Check sheet for the modelled part. Datum: model origin and axes. Units: mm. Face numbers are marked on the shaded views. A direction names the side the tool comes from. Give positions to 0.01 mm unless a question says otherwise; leave off trailing zeros. Order: outer loops, then holes, each group sorted by start corner. A loop starts at its lowest first (then second) coordinate and runs counter-clockwise, first axis right, second up. Notation, with made-up numbers: M -30.75,27 L -10.75,27 A21 cw -10.75,51 Z; hole C -17.5,-29.75 d2. An arc over 180 degrees is marked long. One line per question, with ' | ' between items. Start each with the question number.
```python
from build123d import *

# Parameters (mm, degrees)
BOSS_EXTRUDE1_DEPTH   = 19.812
SKETCH2_R             = 7.62
BOSS_EXTRUDE2_DEPTH   = 14.986
BOSS_EXTRUDE3_DEPTH   = 19.812
CHAMFER1_SIZE2        = 1.397459912
CHAMFER1_SIZE         = 1.361150227
CHAMFER1_EDGE_2_SIZE2 = 1.397459912
CHAMFER1_EDGE_2_SIZE  = 1.361150227


with BuildPart() as part:
    # Sketch1 → Boss-Extrude1 (new body)
    with BuildSketch(Plane(origin=(0, 0, 0), x_dir=(0, -1, 0), z_dir=(-1, 0, 0))):
        Polygon((-9.525, 5.499261314), (-9.525, -5.499261314), (0, -10.998522628), (9.525, -5.499261314), (9.525, 5.499261314), (0, 10.998522628), align=None)
    extrude(amount=-BOSS_EXTRUDE1_DEPTH)

    # Sketch2 → Boss-Extrude2 (add)
    with BuildSketch(Plane(origin=(19.812, 0, 0), x_dir=(0, 0, -1), z_dir=(1, 0, 0))):
        Circle(SKETCH2_R)
    extrude(amount=BOSS_EXTRUDE2_DEPTH)

    # Sketch3 → Boss-Extrude3 (add)
    with BuildSketch(Plane(origin=(34.798, 0, 0), x_dir=(0, -1, 0), z_dir=(-1, 0, 0))):
        Polygon((9.525, -5.499261314), (9.525, 5.499261314), (0, 10.998522628), (-9.525, 5.499261314), (-9.525, -5.499261314), (0, -10.998522628), align=None)
    extrude(amount=-BOSS_EXTRUDE3_DEPTH)

    # Sketch4 → Hole1 (revolve, cut)
    with BuildSketch(Plane(origin=(54.61, 0, 0), x_dir=(0, 0, -1), z_dir=(0, 1, 0))):
        Polygon((0, 0), (0, 9.906), (5.49664229, 9.906), (5.750849773, 0), align=None)
    revolve(axis=Axis((-55.39, 0, 0), (1, 0, 0)), mode=Mode.SUBTRACT)

    # Sketch6 → Hole2 (revolve, cut)
    with BuildSketch(Plane.ZX):
        Polygon((0, 0), (0, 9.906), (5.49664229, 9.906), (5.750849773, 0), align=None)
    revolve(axis=Axis((110, 0, 0), (-1, 0, 0)), mode=Mode.SUBTRACT)

    # Chamfer1
    chamfer1_edges = [part.edges().sort_by_distance(p)[0] for p in [
        (54.61, 0, 5.750849773),
    ]]
    chamfer(chamfer1_edges, length=CHAMFER1_SIZE, length2=CHAMFER1_SIZE2)

    # Chamfer1 edge 2
    chamfer1_edge_2_edges = [part.edges().sort_by_distance(p)[0] for p in [
        (0, 0, -5.750849773),
    ]]
    chamfer(chamfer1_edge_2_edges, length=CHAMFER1_EDGE_2_SIZE, length2=CHAMFER1_EDGE_2_SIZE2)


solid = part.part
```
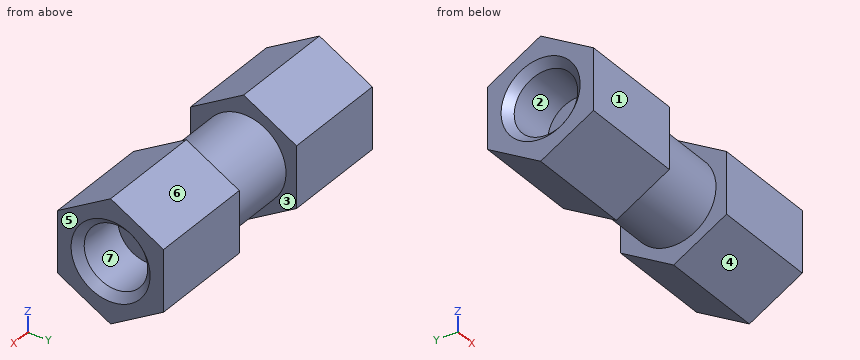
Item 1: Set-up check for the marked faces 1, 2 and 3: record each of +Z, -Z, +X, -X, +Y, -Y from which the full face is reachable in a straight line by a thin tool's end or side.
Item 2: Draft check along Z on the marked faces 4, 5, 6 and 7. Enter one of: released by +Z, released by -Z, zero draft, split by the parting line, or undercut.
Item 3: Go/stop test with flat-tipped pins: P1, Ø9, axis at y = -1.5, z = 1, coming from the -X side; P2, Ø3.5, axis at y = -0.5, z = 2, coming from the +X side; P3, Ø1.5, axis at x = 23.5, y = -3, coming from the -Z side. Record where each tip stops, or that it passes through.
Item 4: Section check D-D, the plane z = 8.5. Record the cut outline in (x, y).
Item 5: Section check A-A, the plane z = 0. Record the cut outline in (x, y) (3 decimals), then the cut area to 3 significant figures.
Item 6: Scan lines: probe 1 along X at (y, z) = (1.5, 10); probe 2 along Y at (x, z) = (47, -0.75) (3 decimals); probe 3 along Z at (x, y) = (51, 1). Record each from-to range of solid material in increasing order. Write a range as [from, to].
Item 7: Section check B-B, the plane y = 8.25. Record the cut outline in (x, z), then the cut area to 3 significant figures.
Item 8: Section check C-C, the plane x = 17. Record the cut outline in (y, z) (3 decimals).
Reported:
1) face 1: +Z, -Z, +X, -X, -Y | face 2: -X | face 3: none
2) face 4: released by -Z | face 5: zero draft | face 6: released by +Z | face 7: undercut
3) P1: stops at x = 0.81 | P2: stops at x = 44.7 | P3: stops at z = -7.28
4) outline: M 0,-4.33 L 19.81,-4.33 L 19.81,4.33 L 0,4.33 Z; M 34.8,-4.33 L 54.61,-4.33 L 54.61,4.33 L 34.8,4.33 Z
5) outline: M 0,-9.525 L 19.812,-9.525 L 19.812,-7.62 L 34.798,-7.62 L 34.798,-9.525 L 54.61,-9.525 L 54.61,-7.112 L 53.213,-5.715 L 44.704,-5.497 L 44.704,5.497 L 53.213,5.715 L 54.61,7.112 L 54.61,9.525 L 34.798,9.525 L 34.798,7.62 L 19.812,7.62 L 19.812,9.525 L 0,9.525 L 0,7.112 L 1.397,5.715 L 9.906,5.497 L 9.906,-5.497 L 1.397,-5.715 L 0,-7.112 Z | area: 757 mm^2
6) probe 1: x = [0, 19.81], [34.8, 54.61] | probe 2: y = [-9.525, -5.505], [5.505, 9.525] | probe 3: z = [-10.42, -5.57], [5.57, 10.42]
7) outline: M 0,-6.24 L 19.81,-6.24 L 19.81,6.24 L 0,6.24 Z; M 34.8,-6.24 L 54.61,-6.24 L 54.61,6.24 L 34.8,6.24 Z | area: 494 mm^2
8) outline: M -9.525,-5.499 L 0,-10.999 L 9.525,-5.499 L 9.525,5.499 L 0,10.999 L -9.525,5.499 Z
